from build123d import *

# Parameters (mm, degrees)
BOSS_EXTRUDE1_DEPTH        = 48
F_4_1_4_1_DIAMETER_HOLE1_D = 4.1
LPATTERN1_COUNT            = 6
LPATTERN1_PITCH            = 8
LPATTERN1_COUNT_DIR2       = 3
LPATTERN1_PITCH_DIR2       = 8
MIRROR1_COPY_1_D           = 4.1
MIRROR1_COPY_2_D           = 4.1
MIRROR1_COPY_3_D           = 4.1
MIRROR1_COPY_4_D           = 4.1
MIRROR1_COPY_5_D           = 4.1
MIRROR1_COPY_6_D           = 4.1
MIRROR1_COPY_7_D           = 4.1
MIRROR1_COPY_8_D           = 4.1
MIRROR1_COPY_9_D           = 4.1
MIRROR1_COPY_10_D          = 4.1
MIRROR1_COPY_11_D          = 4.1
MIRROR1_COPY_12_D          = 4.1
MIRROR1_COPY_13_D          = 4.1
MIRROR1_COPY_14_D          = 4.1
MIRROR1_COPY_15_D          = 4.1
MIRROR1_COPY_16_D          = 4.1
MIRROR1_COPY_17_D          = 4.1


with BuildPart() as part:
    # Sketch3 → Boss-Extrude1 (new body)
    with BuildSketch(Plane(origin=(0, 0, 0), x_dir=(0, 0, -1), z_dir=(1, 0, 0))):
        Polygon((0, 0), (0, 26), (-2, 26), (-2, 2), (-26, 2), (-26, 0), align=None)
    extrude(amount=BOSS_EXTRUDE1_DEPTH)

    # Ø4.1 (4.1) Diameter Hole1 (through all)
    with Locations(Plane.XY.offset(2)):
        with Locations((4, 22)):
            f_4_1_4_1_diameter_hole1 = Hole(F_4_1_4_1_DIAMETER_HOLE1_D / 2)

    # LPattern1: 4.1 _4.1_ Diameter Hole1 6 × 3
    with Locations(*[(i * LPATTERN1_PITCH, -j * LPATTERN1_PITCH_DIR2, 0) for i in range(LPATTERN1_COUNT) for j in range(LPATTERN1_COUNT_DIR2) if (i, j) != (0, 0)]):
        add(f_4_1_4_1_diameter_hole1, mode=Mode.SUBTRACT)

    # Mirror1: Ø4.1 (4.1) Diameter Hole1 across plane
    add(f_4_1_4_1_diameter_hole1.mirror(Plane(origin=(0, 0, 0), x_dir=(0, 0.7071067811865471, 0.7071067811865479), z_dir=(0, -0.7071067811865479, 0.7071067811865471))), mode=Mode.SUBTRACT)

    # Mirror1 copy 1 (through all)
    with Locations(Plane(origin=(0, 2, -8), x_dir=(1, 0, 0), z_dir=(0, 1, 0))):
        with Locations((4, -22)):
            Hole(MIRROR1_COPY_1_D / 2)

    # Mirror1 copy 2 (through all)
    with Locations(Plane(origin=(0, 2, -16), x_dir=(1, 0, 0), z_dir=(0, 1, 0))):
        with Locations((4, -22)):
            Hole(MIRROR1_COPY_2_D / 2)

    # Mirror1 copy 3 (through all)
    with Locations(Plane(origin=(8, 2, 0), x_dir=(1, 0, 0), z_dir=(0, 1, 0))):
        with Locations((4, -22)):
            Hole(MIRROR1_COPY_3_D / 2)

    # Mirror1 copy 4 (through all)
    with Locations(Plane(origin=(8, 2, -8), x_dir=(1, 0, 0), z_dir=(0, 1, 0))):
        with Locations((4, -22)):
            Hole(MIRROR1_COPY_4_D / 2)

    # Mirror1 copy 5 (through all)
    with Locations(Plane(origin=(8, 2, -16), x_dir=(1, 0, 0), z_dir=(0, 1, 0))):
        with Locations((4, -22)):
            Hole(MIRROR1_COPY_5_D / 2)

    # Mirror1 copy 6 (through all)
    with Locations(Plane(origin=(16, 2, 0), x_dir=(1, 0, 0), z_dir=(0, 1, 0))):
        with Locations((4, -22)):
            Hole(MIRROR1_COPY_6_D / 2)

    # Mirror1 copy 7 (through all)
    with Locations(Plane(origin=(16, 2, -8), x_dir=(1, 0, 0), z_dir=(0, 1, 0))):
        with Locations((4, -22)):
            Hole(MIRROR1_COPY_7_D / 2)

    # Mirror1 copy 8 (through all)
    with Locations(Plane(origin=(16, 2, -16), x_dir=(1, 0, 0), z_dir=(0, 1, 0))):
        with Locations((4, -22)):
            Hole(MIRROR1_COPY_8_D / 2)

    # Mirror1 copy 9 (through all)
    with Locations(Plane(origin=(24, 2, 0), x_dir=(1, 0, 0), z_dir=(0, 1, 0))):
        with Locations((4, -22)):
            Hole(MIRROR1_COPY_9_D / 2)

    # Mirror1 copy 10 (through all)
    with Locations(Plane(origin=(24, 2, -8), x_dir=(1, 0, 0), z_dir=(0, 1, 0))):
        with Locations((4, -22)):
            Hole(MIRROR1_COPY_10_D / 2)

    # Mirror1 copy 11 (through all)
    with Locations(Plane(origin=(24, 2, -16), x_dir=(1, 0, 0), z_dir=(0, 1, 0))):
        with Locations((4, -22)):
            Hole(MIRROR1_COPY_11_D / 2)

    # Mirror1 copy 12 (through all)
    with Locations(Plane(origin=(32, 2, 0), x_dir=(1, 0, 0), z_dir=(0, 1, 0))):
        with Locations((4, -22)):
            Hole(MIRROR1_COPY_12_D / 2)

    # Mirror1 copy 13 (through all)
    with Locations(Plane(origin=(32, 2, -8), x_dir=(1, 0, 0), z_dir=(0, 1, 0))):
        with Locations((4, -22)):
            Hole(MIRROR1_COPY_13_D / 2)

    # Mirror1 copy 14 (through all)
    with Locations(Plane(origin=(32, 2, -16), x_dir=(1, 0, 0), z_dir=(0, 1, 0))):
        with Locations((4, -22)):
            Hole(MIRROR1_COPY_14_D / 2)

    # Mirror1 copy 15 (through all)
    with Locations(Plane(origin=(40, 2, 0), x_dir=(1, 0, 0), z_dir=(0, 1, 0))):
        with Locations((4, -22)):
            Hole(MIRROR1_COPY_15_D / 2)

    # Mirror1 copy 16 (through all)
    with Locations(Plane(origin=(40, 2, -8), x_dir=(1, 0, 0), z_dir=(0, 1, 0))):
        with Locations((4, -22)):
            Hole(MIRROR1_COPY_16_D / 2)

    # Mirror1 copy 17 (through all)
    with Locations(Plane(origin=(40, 2, -16), x_dir=(1, 0, 0), z_dir=(0, 1, 0))):
        with Locations((4, -22)):
            Hole(MIRROR1_COPY_17_D / 2)


solid = part.part
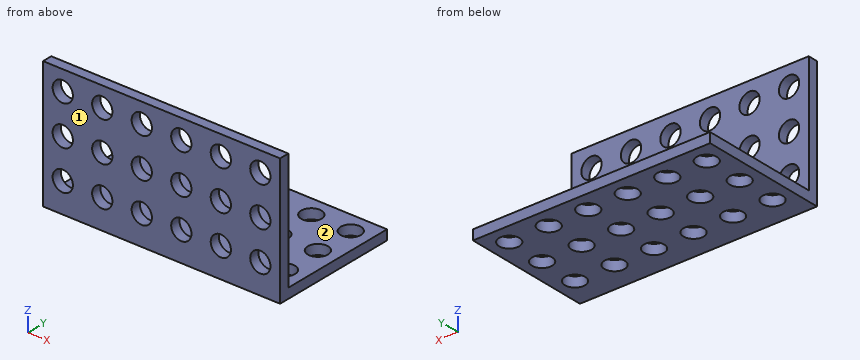
The listing builds one solid part. Answer for the finished solid, in the listing's coordinates (mm). Face numbers are marked on the shaded views. A direction names the side the tool comes from. Give positions to 0.01 mm unless a question says otherwise; leave off trailing zeros. Write each loop counter-clockwise with the first axis right and the second up, starting at its lowest first coordinate (ties: lowest second). Pieces come first, ordered by that corner, then holes. Notation, with made-up numbers: (-30.75, 62) - (-12.75, 62) arc R6 ccw to (-12.75, 67) - close; hole circle Ø8 at (7.25, 64.25). An arc over 180 degrees is marked (long way). One line per question, with ' | ' between items. Start each with the question number.
1. Given P1, Ø3.5, axis at x = 44, z = 6, coming from the +Y side; P2, Ø5.5, axis at x = 36, z = 14, coming from the +Y side; P3, Ø4.5, axis at x = 20, z = 14, coming from the -Y side; P4, Ø12, axis at x = 39.5, y = 15.5, coming from the +Z side, each flat-ended and moving along its own axis, determine where each tip first touches the part or whether it passes through.
2. For the marked faces 1 and 2, determine the directions among +Z, -Z, +X, -X, +Y, -Y from which every point of the face is accessible in a straight line to the end or side of a thin tool.
3. Section A-A, the plane y = 22 is taken. Determine the outline of the cut face in (x, z).
4. Straight lines are drawn through the part: line 1 (Z direction, x = 36, y = 0.7); line 2 (Y direction, x = 5.5, z = 8). For each, find the intervals that lie inside material, in ascending order.
5. Section B-B, the plane x = 4 is taken. Count the separate pieces of the cut face and the enclosed holes in it, then the cut area to 3 significant figures.
Result:
1) P1: passes through | P2: stops at y = 2 | P3: stops at y = 0 | P4: stops at z = 2
2) face 1: +Z, -Z, +X, -X, -Y | face 2: +Z, +X, -X, +Y
3) outline: (0, 0) - (1.95, 0) - (1.95, 2) - (0, 2) - close; (6.05, 0) - (9.95, 0) - (9.95, 2) - (6.05, 2) - close; (14.05, 0) - (17.95, 0) - (17.95, 2) - (14.05, 2) - close; (22.05, 0) - (25.95, 0) - (25.95, 2) - (22.05, 2) - close; (30.05, 0) - (33.95, 0) - (33.95, 2) - (30.05, 2) - close; (38.05, 0) - (41.95, 0) - (41.95, 2) - (38.05, 2) - close; (46.05, 0) - (48, 0) - (48, 2) - (46.05, 2) - close
4) line 1: z = 0 to 3.95, 8.05 to 11.95, 16.05 to 19.95, 24.05 to 26 | line 2: y = 0 to 2
5) separate pieces: 7 | enclosed holes: 0 | area: 50.8 mm2
